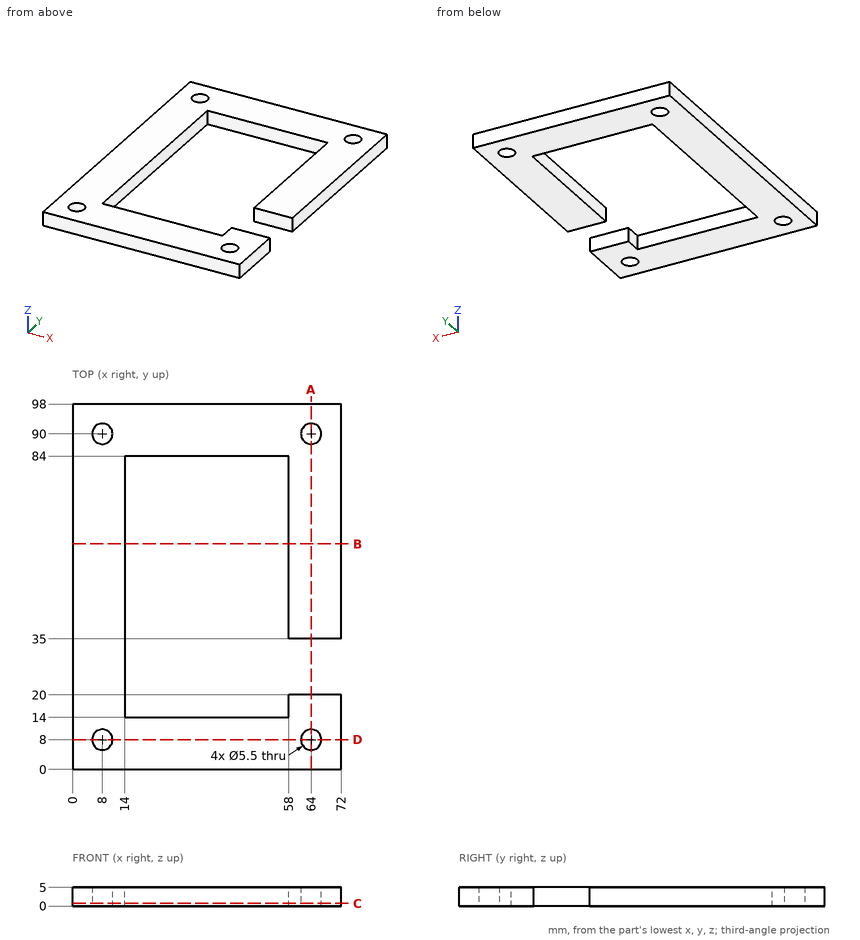
Verification items for this drawing (mm, ordinates from the low corner). Coordinates: 2 decimals unless noted, no trailing zeros. Write each loop counter-clockwise with the first axis right and the second up, starting at its lowest first coordinate (ties: lowest second). Pieces come first, ordered by that corner, then holes. Notation, with made-up numbers: M -12,54.5 L 13,54.5 A5 ccw 13,61.5 Z; hole C -28.5,11.5 d6. An arc over 180 degrees is marked long. Answer as CSV lines item,"result".
Q1. Cross-section at C-C (z = 0.75). Record the boundary of the cut face in (x, y), then the cut area to 3 significant figures.
Check result:
outline,"M 0,0 L 72,0 L 72,20 L 58,20 L 58,14 L 14,14 L 14,84 L 58,84 L 58,35 L 72,35 L 72,98 L 0,98 Z; hole C 8,8 d5.5; hole C 8,90 d5.5; hole C 64,8 d5.5; hole C 64,90 d5.5"
area,"3,670 mm^2"
Q2. Cross-section at B-B (y = 60.5). Record the boundary of the cut face in (x, z), then the cut area to 3 significant figures.
Check result:
outline,"M 0,0 L 14,0 L 14,5 L 0,5 Z; M 58,0 L 72,0 L 72,5 L 58,5 Z"
area,"140 mm^2"
Q3. Material ranges on probe 1 along Y at (x, z) = (8, 4.05); probe 2 along Y at (x, z) = (64, 2.85); probe 3 along Y at (x, z) = (49, 4.75), recorded low to high. Write a range as from..to.
Check result:
probe 1,"0..5.25, 10.75..87.25, 92.75..98"
probe 2,"0..5.25, 10.75..20, 35..87.25, 92.75..98"
probe 3,"0..14, 84..98"
Q4. Cross-section at A-A (x = 64). Record the boundary of the cut face in (y, z), then the cut area to 3 significant figures.
Check result:
outline,"M 0,0 L 5.25,0 L 5.25,5 L 0,5 Z; M 10.75,0 L 20,0 L 20,5 L 10.75,5 Z; M 35,0 L 87.25,0 L 87.25,5 L 35,5 Z; M 92.75,0 L 98,0 L 98,5 L 92.75,5 Z"
area,"360 mm^2"
Q5. Go/stop test with a flat-tipped pin: pin 1 (1.5 mm diameter, centred on y = 34, z = 3, fed in from +X). Record where the tip stops, or that it passes through.
Check result:
pin 1,"x = 14"
Q6. Cross-section at D-D (y = 8). Record the boundary of the cut face in (x, z).
Check result:
outline,"M 0,0 L 5.25,0 L 5.25,5 L 0,5 Z; M 10.75,0 L 61.25,0 L 61.25,5 L 10.75,5 Z; M 66.75,0 L 72,0 L 72,5 L 66.75,5 Z"
